For this review, take the finished solid that the model builds, in its own axes (mm). Face numbers are marked on the shaded views. Round coordinates to 2 decimals unless told otherwise and drop trailing zeros. Loops run counter-clockwise (first coordinate to the right, second up) from the corner with the lowest first, then second, coordinate; pieces in that order, holes last. Notation, with made-up numbers: M 40,14 L 89,14 A14 cw 89,39 Z; hole C 4,0.5 d1. An arc over 180 degrees is marked long. One line per question, with ' | ' between items. Start each with the question number.
1) We need section A-A (z = 0). Give the boundary of the cut face in (x, y).
2) We need section C-C (y = 2.7). Give the boundary of the cut face in (x, z), and give its area (3 significant figures).
3) For probe 1 along X at (y, z) = (2.95, 0); probe 2 along Y at (x, z) = (1, 3.25); probe 3 along Z at (x, y) = (1.5, 0.7), list the stretches that pass through material, from the lowest coordinate up. Write a range as from..to.
4) We need section B-B (x = 0). Give the boundary of the cut face in (y, z), and give its area (3 significant figures).
5) Mouldability with a two-part tool opening along Z and no side actions: class the marked faces 1, 2 and 3 as pulls with the +Z half, pulls with the -Z half, needs draft (parallel to the pull), parting line crosses it, or undercut.
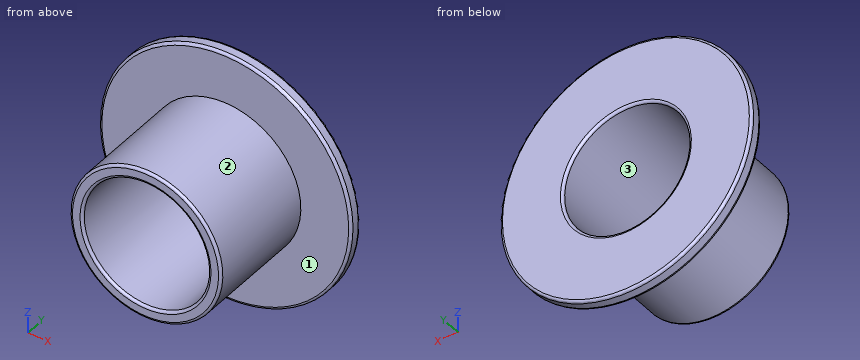
```python
from build123d import *

# Parameters (mm, degrees)
SKETCH1_R           = 3
SKETCH1_R_2         = 2.5
BOSS_EXTRUDE1_DEPTH = 4.5
SKETCH2_R           = 5
SKETCH2_R_2         = 2.5
BOSS_EXTRUDE2_DEPTH = 0.5
FILLET1_R           = 0.1


with BuildPart() as part:
    # Sketch1 → Boss-Extrude1 (new body)
    with BuildSketch(Plane(origin=(0, 0, 0), x_dir=(1, 0, 0), z_dir=(0, 1, 0))):
        with Locations(Location((0, 0, 0), (0, 0, 270))):
            Circle(SKETCH1_R)
        with Locations(Location((0, 0, 0), (0, 0, 270))):
            Circle(SKETCH1_R_2, mode=Mode.SUBTRACT)
    extrude(amount=BOSS_EXTRUDE1_DEPTH)

    # Sketch2 → Boss-Extrude2 (add)
    with BuildSketch(Plane(origin=(0, 4.5, 0), x_dir=(1, 0, 0), z_dir=(0, 1, 0))):
        with Locations(Location((0, 0, 0), (0, 0, 270))):
            Circle(SKETCH2_R)
        with Locations(Location((0, 0, 0), (0, 0, 270))):
            Circle(SKETCH2_R_2, mode=Mode.SUBTRACT)
    extrude(amount=BOSS_EXTRUDE2_DEPTH)

    # Fillet1
    fillet1_edges = [part.edges().sort_by_distance(p)[0] for p in [
        (0, 4.5, -5),
        (0, 5, -2.5),
        (0, 0, -3),
        (0, 0, -2.5),
        (0, 5, -5),
    ]]
    fillet(fillet1_edges, radius=FILLET1_R)


solid = part.part
```
Answers below:
1) outline: M -5,4.6 A0.1 ccw -4.9,4.5 L -3,4.5 L -3,0.1 A0.1 ccw -2.9,0 L -2.6,0 A0.1 ccw -2.5,0.1 L -2.5,4.9 A0.1 ccw -2.6,5 L -4.9,5 A0.1 ccw -5,4.9 Z; M 2.5,0.1 A0.1 ccw 2.6,0 L 2.9,0 A0.1 ccw 3,0.1 L 3,4.5 L 4.9,4.5 A0.1 ccw 5,4.6 L 5,4.9 A0.1 ccw 4.9,5 L 2.6,5 A0.1 ccw 2.5,4.9 Z
2) outline: C 0,0 d6; hole C 0,0 d5 | area: 8.64 mm^2
3) probe 1: -3..-2.5, 2.5..3 | probe 2: 4.5..5 | probe 3: -2.6..-2, 2..2.6
4) outline: M 0,-2.9 A0.1 ccw 0.1,-3 L 4.5,-3 L 4.5,-4.9 A0.1 ccw 4.6,-5 L 4.9,-5 A0.1 ccw 5,-4.9 L 5,-2.6 A0.1 ccw 4.9,-2.5 L 0.1,-2.5 A0.1 ccw 0,-2.6 Z; M 0,2.6 A0.1 ccw 0.1,2.5 L 4.9,2.5 A0.1 ccw 5,2.6 L 5,4.9 A0.1 ccw 4.9,5 L 4.6,5 A0.1 ccw 4.5,4.9 L 4.5,3 L 0.1,3 A0.1 ccw 0,2.9 Z | area: 6.98 mm^2
5) face 1: needs draft | face 2: parting line crosses it | face 3: undercut
